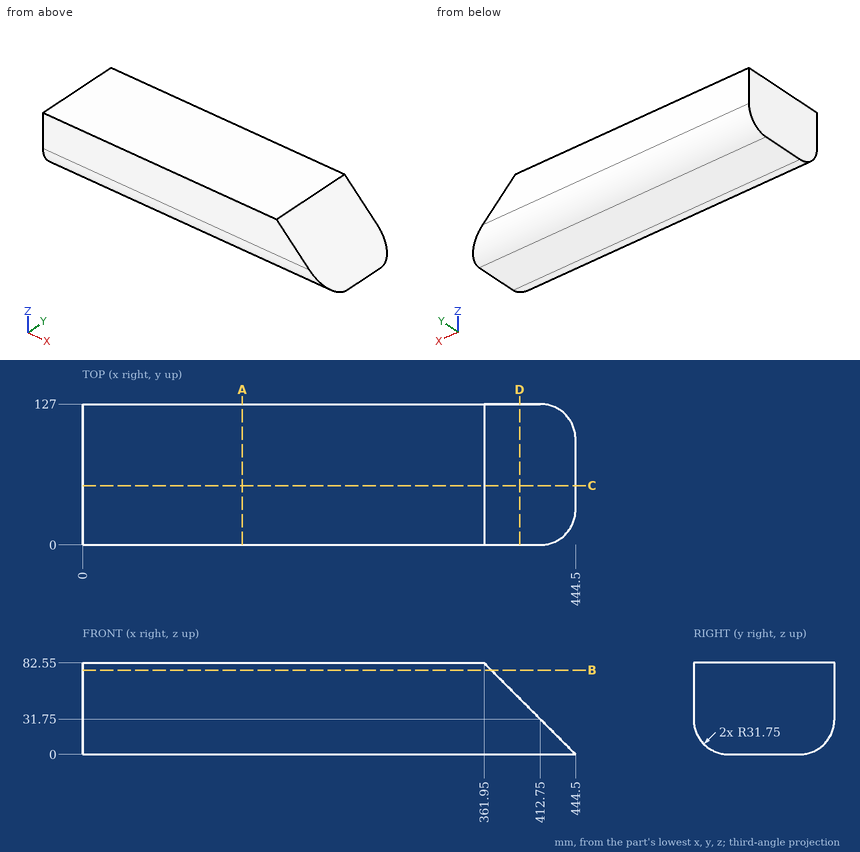
Input: dimensioned drawing with shaded views. Units: mm. Origin: part minimum x, y, z. Give positions to 0.01 mm unless a question says otherwise; leave off trailing zeros. Order: outer loops, then holes, each group sorted by start corner. A loop starts at its lowest first (then second) coordinate and runs counter-clockwise, first axis right, second up. Notation, with made-up numbers: (82.25, 13) -> (134.25, 13) arc R21 cw to (134.25, 23) -> close; hole circle Ø1 at (69.25, 68). An arc over 180 degrees is marked (long way). Write item = value, one per line.
Item 1: Section query A-A (x = 144). Output: boundary loops of the cut face in (y, z), then the cut area to 3 significant figures.
Check result:
outline = (0, 31.75) arc R31.75 ccw to (31.75, 0) -> (95.25, 0) arc R31.75 ccw to (127, 31.75) -> (127, 82.55) -> (0, 82.55) -> close
area = 10,100 mm²
Item 2: Ray query, probe 1 along Z at (x, y) = (388, 76); probe 2 along Z at (x, y) = (311, 10.5); probe 3 along Y at (x, z) = (308, 21.5). Return the intervals inside material, ascending.
Check result:
probe_1 = 0 to 56.5
probe_2 = 8.16 to 82.55
probe_3 = 1.7 to 125.3
Item 3: Contact query for a flat-ended pin moving along its axis: pin 1 (2 mm diameter, centred on y = 21, z = 16, fed in from +X). Output: stop coordinate, or through.
Check result:
pin_1 = 429.5
Item 4: Section query C-C (y = 53.5). Output: boundary loops of the cut face in (x, z), then the cut area to 3 significant figures.
Check result:
outline = (0, 0) -> (444.5, 0) -> (361.95, 82.55) -> (0, 82.55) -> close
area = 33,300 mm²
Item 5: Section query B-B (z = 76). Output: boundary loops of the cut face in (x, y).
Check result:
outline = (0, 0) -> (368.5, 0) -> (368.5, 127) -> (0, 127) -> close
Item 6: Section query D-D (x = 394). Output: boundary loops of the cut face in (y, z), then the cut area to 3 significant figures.
Check result:
outline = (0, 31.75) arc R31.75 ccw to (31.75, 0) -> (95.25, 0) arc R31.75 ccw to (127, 31.75) -> (127, 50.5) -> (0, 50.5) -> close
area = 5,980 mm²
